The listing builds one solid part. Answer for the finished solid, in the listing's coordinates (mm). Face numbers are marked on the shaded views. A direction names the side the tool comes from. Give positions to 0.01 mm unless a question says otherwise; leave off trailing zeros. Loops run counter-clockwise (first coordinate to the right, second up) from the corner with the lowest first, then second, coordinate; pieces in that order, holes last. Notation, with made-up numbers: M 51.25,18.25 L 72.25,18.25 A21 ccw 72.25,35.25 Z; hole C -1,-22 d6. An arc over 180 degrees is marked long. One line per item, written item: value. Start each with the question number.
Q1. A flat-ended cylindrical pin translates along its axis: pin 1 (8 mm diameter, centred on x = 57.5, y = 0, fed in from +Z). Find the tip coordinate at first contact, or state that the pin passes through.
Q2. A cutting plane is placed at A-A, the plane z = 14. Determine the outline of the cut face in (x, y).
Q3. A cutting plane is placed at C-C, the plane y = 0. Determine the outline of the cut face in (x, z).
Q4. For the marked faces 5, 6 and 7, determine the directions among +Z, -Z, +X, -X, +Y, -Y from which every point of the face is accessible in a straight line to the end or side of a thin tool.
Q5. A cutting plane is placed at D-D, the plane y = 26.5. Determine the outline of the cut face in (x, z).
Q6. Consider L1, parallel to Y at x = -35, z = 2; L2, parallel to Z at x = -33, y = -10.5; L3, parallel to X at y = 26, z = 21.5. Determine where each line is inside the solid, lowest interval first.
Q7. A cutting plane is placed at B-B, the plane x = 57.5. Determine the outline of the cut face in (y, z), and give its area (3 significant figures).
Q8. The mould has two halves that part along Y. Classify the marked faces 1, 2, 3 and 4: +Y half, -Y half, draft (parallel to the pull), parting line (faces both ways), or undercut.
from build123d import *

# Parameters (mm, degrees)
F0_W           = 130
F0_H           = 60
F1_DEPTH       = 10.6
F2_W           = 14.75
F2_H           = 10
F3_DEPTH       = 20
F5_D           = 6.8
F7_D           = 6
F7_CSINK_D     = 17
F7_CSINK_ANGLE = 90
F8_SIZE        = 1


with BuildPart() as f1:
    # F0 (on Top) → F1 (new body)
    with BuildSketch(Plane.XY):
        Rectangle(F0_W, F0_H)
    extrude(amount=F1_DEPTH)

    # F2 (on face) → F3 (join)
    with BuildSketch(Plane.XY.offset(10.6)):
        with Locations((-57.625, 25)):
            Rectangle(F2_W, F2_H)
        with Locations((-57.625, -25)):
            Rectangle(F2_W, F2_H)
        with Locations((57.625, -25)):
            Rectangle(F2_W, F2_H)
        with Locations((57.625, 25)):
            Rectangle(F2_W, F2_H)
    extrude(amount=F3_DEPTH)

    # F5 (through all)
    with Locations(Plane.XY.offset(10.6)):
        with Locations((57.5, 0), (-57.5, 0)):
            Hole(F5_D / 2)

    # F7 (through all)
    with Locations(Plane.XY.offset(10.6)):
        with Locations((35, 0), (-35, 0)):
            CounterSinkHole(F7_D / 2, F7_CSINK_D / 2, counter_sink_angle=F7_CSINK_ANGLE)

    # F8
    f8_edges = [f1.edges().sort_by_distance(p)[0] for p in [
        (-57.625, -30, 30.6),
        (-50.25, -25, 30.6),
        (-57.625, -20, 30.6),
        (-65, -25, 30.6),
        (-57.625, 20, 30.6),
        (-57.625, 30, 30.6),
        (-50.25, 25, 30.6),
        (-65, 25, 30.6),
        (50.25, -25, 30.6),
        (57.625, -20, 30.6),
        (65, -25, 30.6),
        (57.625, -30, 30.6),
        (65, 25, 30.6),
        (57.625, 20, 30.6),
        (50.25, 25, 30.6),
        (57.625, 30, 30.6),
    ]]
    chamfer(f8_edges, length=F8_SIZE)


solid = f1.part
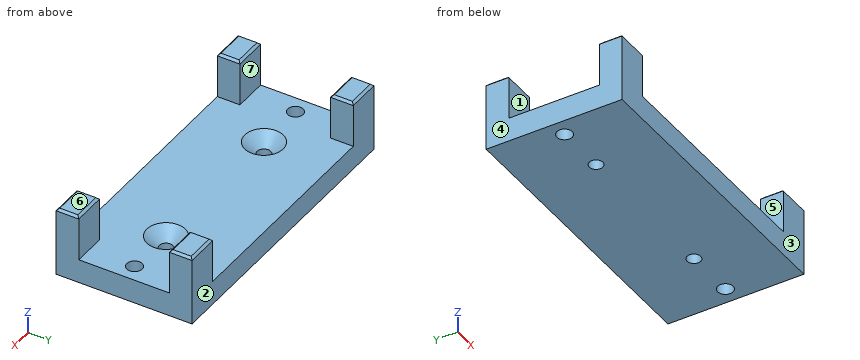
Answer block:
1. pin 1: z = 10.6
2. outline: M -65,-30 L -50.25,-30 L -50.25,-20 L -65,-20 Z; M -65,20 L -50.25,20 L -50.25,30 L -65,30 Z; M 50.25,-30 L 65,-30 L 65,-20 L 50.25,-20 Z; M 50.25,20 L 65,20 L 65,30 L 50.25,30 Z
3. outline: M -65,0 L -60.9,0 L -60.9,10.6 L -65,10.6 Z; M -54.1,0 L -38,0 L -38,5.1 L -43.5,10.6 L -54.1,10.6 Z; M -32,0 L 32,0 L 32,5.1 L 26.5,10.6 L -26.5,10.6 L -32,5.1 Z; M 38,0 L 54.1,0 L 54.1,10.6 L 43.5,10.6 L 38,5.1 Z; M 60.9,0 L 65,0 L 65,10.6 L 60.9,10.6 Z
4. face 5: +Z, +Y, -Y
4. face 6: +Z, +X, -X, +Y, -Y
4. face 7: +Z, +X, -X
5. outline: M -65,0 L 65,0 L 65,29.6 L 64,30.6 L 51.25,30.6 L 50.25,29.6 L 50.25,10.6 L -50.25,10.6 L -50.25,29.6 L -51.25,30.6 L -64,30.6 L -65,29.6 Z
6. L1: -30 to -3, 3 to 30
6. L2: 0 to 10.6
6. L3: -65 to -50.25, 50.25 to 65
7. outline: M -30,0 L -3.4,0 L -3.4,10.6 L -20,10.6 L -20,29.6 L -21,30.6 L -29,30.6 L -30,29.6 Z; M 3.4,0 L 30,0 L 30,29.6 L 29,30.6 L 21,30.6 L 20,29.6 L 20,10.6 L 3.4,10.6 Z
7. area: 962 mm^2
8. face 1: undercut
8. face 2: +Y half
8. face 3: -Y half
8. face 4: draft
